Work out the finished part from the listing and answer in its coordinate system (mm). A direction names the side the tool comes from. Round coordinates to 2 decimals unless told otherwise and drop trailing zeros. Order: outer loops, then holes, each group sorted by start corner. A loop starts at its lowest first (then second) coordinate and runs counter-clockwise, first axis right, second up. Notation, with made-up numbers: (68.25, 37) - (106.25, 37) arc R4 cw to (106.25, 44) - close; hole circle Ø11 at (-22.75, 11.25). An arc over 180 degrees is marked (long way). Put each result on its own line as item: value.
```python
from build123d import *

# Parameters (mm, degrees)
SKETCH1_W           = 95
SKETCH1_H           = 95
SKETCH1_R           = 37.5
BOSS_EXTRUDE1_DEPTH = 2
SKETCH3_W           = 10
SKETCH3_H           = 4
SKETCH3_W_2         = 9
CUT_EXTRUDE5_DEPTH  = 68.294130502
FILLET1_R           = 5


with BuildPart() as part:
    # Sketch1 → Boss-Extrude1 (new, symmetric)
    with BuildSketch(Plane(origin=(0, 0, 0), x_dir=(1, 0, 0), z_dir=(0, 1, 0))):
        Rectangle(SKETCH1_W, SKETCH1_H)
        with Locations(Location((0, 0, 0), (0, 0, 270))):
            Circle(SKETCH1_R, mode=Mode.SUBTRACT)
    extrude(amount=BOSS_EXTRUDE1_DEPTH, both=True)

    # Sketch3 → Cut-Extrude5 (cut, through all)
    with BuildSketch(Plane(origin=(0, 2, 0), x_dir=(1, 0, 0), z_dir=(0, 1, 0))):
        with Locations((-42.5, 37.5)):
            Rectangle(SKETCH3_W, SKETCH3_H)
        with Locations((-21, 37.5)):
            Rectangle(SKETCH3_W_2, SKETCH3_H)
        with Locations((21, 37.5)):
            Rectangle(SKETCH3_W_2, SKETCH3_H)
        with Locations((42.5, 37.5)):
            Rectangle(SKETCH3_W, SKETCH3_H)
        with Locations((42.5, -37.5)):
            Rectangle(SKETCH3_W, SKETCH3_H)
        with Locations((21, -37.5)):
            Rectangle(SKETCH3_W_2, SKETCH3_H)
        with Locations((-21, -37.5)):
            Rectangle(SKETCH3_W_2, SKETCH3_H)
        with Locations((-42.5, -37.5)):
            Rectangle(SKETCH3_W, SKETCH3_H)
    extrude(amount=-CUT_EXTRUDE5_DEPTH, mode=Mode.SUBTRACT)

    # Fillet1
    fillet1_edges = [part.edges().sort_by_distance(p)[0] for p in [
        (47.5, 0, 47.5),
        (-47.5, 0, 47.5),
        (-47.5, 0, -47.5),
        (47.5, 0, -47.5),
    ]]
    fillet(fillet1_edges, radius=FILLET1_R)


solid = part.part
```
1) For a pull along Z with two mould halves and no side action, classify faces 1 (the flat face through (-1, 0, 47.5)), 2 (the cylindrical face through (-46.07, -0.03, -46)), 3 (the flat face through (-43, 0, 39.5)) as pulls with the +Z half, pulls with the -Z half, needs draft (parallel to the pull), parting line crosses it, or undercut.
Findings below:
face 1: pulls with the +Z half
face 2: pulls with the -Z half
face 3: undercut
2) A cutting plane is placed at C-C on y = -1.3. Give the number of separate pieces and of enclosed holes in the cut face, then the cut area to 3 significant figures.
Findings below:
separate pieces: 1
enclosed holes: 5
area: 4,280 mm2
3) A cutting plane is placed at B-B on x = 0. Write down the section's boundary in (y, z).
Findings below:
outline: (-2, -47.5) - (2, -47.5) - (2, -37.5) - (-2, -37.5) - close; (-2, 37.5) - (2, 37.5) - (2, 47.5) - (-2, 47.5) - close
4) A cutting plane is placed at A-A on z = 0. Write down the section's boundary in (x, y).
Findings below:
outline: (-47.5, -2) - (-37.5, -2) - (-37.5, 2) - (-47.5, 2) - close; (37.5, -2) - (47.5, -2) - (47.5, 2) - (37.5, 2) - close
5) Given pin 1 Ø2 at (x, y) = (43, -0.5) entering from -Z; pin 2 Ø2 at (y, z) = (1, -38) entering from +X; pin 3 Ø2 at (y, z) = (0.5, 38) entering from -X, each flat-ended and moving along its own axis, determine where each tip first touches the part or whether it passes through.
Findings below:
pin 1: stops at z = -47.5
pin 2: stops at x = 37.5
pin 3: stops at x = -37.5
6) Straight lines are drawn through the part: L1, parallel to Z at x = -42, y = 1.6; L2, parallel to Z at x = -0.5, y = -0.5. For each, find the intervals that lie inside material, in ascending order. Write a range as from..to.
Findings below:
L1: z = -47.5..-39.5, -35.5..35.5, 39.5..47.5
L2: z = -47.5..-37.5, 37.5..47.5
7) For faces 4 (the flat face through (-43, 0, -39.5)), 5 (the flat face through (16.5, 0, 38)), 6 (the cylindrical face through (46, 0.03, 46.07)), 7 (the cylindrical face through (-46.07, 0.03, 46)), 8 (the flat face through (37.5, 0, 38)), determine the directions among +Z, -Z, +X, -X, +Y, -Y from which every point of the face is accessible in a straight line to the end or side of a thin tool.
Findings below:
face 4: -X, +Y, -Y
face 5: +Y, -Y
face 6: +Z, +X, +Y, -Y
face 7: +Z, -X, +Y, -Y
face 8: +X, +Y, -Y
